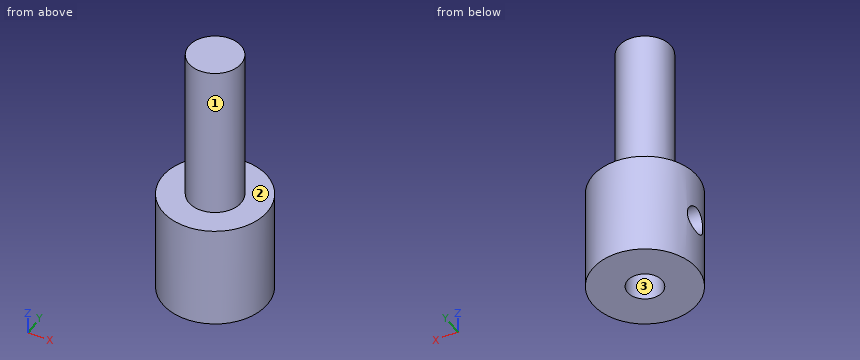
Autodesk Inventor part; units mm, degrees
ref_plane "YZ Plane" through (0, 0, 0) normal (1, 0, 0) x (0, 1, 0)
ref_plane "XZ Plane" through (0, 0, 0) normal (0, 1, 0) x (-1, 0, 0)
ref_plane "XY Plane" through (0, 0, 0) normal (0, 0, 1) x (1, 0, 0)
sketch "スケッチ1" plane through (0, 0, 0) normal (1, 0, 0) x (0, 1, 0)
  line L0 (0, 0) -> (1.5, 0)
  line L1 (1.5, 0) -> (1.5, -9)
  line L2 (1.5, -9) -> (3, -9)
  line L3 (3, -9) -> (3, -15)
  line L4 (3, -15) -> (1, -15)
  line L5 (0, 0) -> (0, -11)
  line L6 (0, -11) -> (1, -11)
  line L7 (1, -11) -> (1, -15)
  dimension "d0" = 1.5
  dimension "d1" = 1
  dimension "d2" = 9
  dimension "d3" = 4
  dimension "d4" = 2
  dimension "d5" = 2
revolve "回転1" add sketch "スケッチ1" angle 360 about axis through (0, 0, 0) along (0, 0, -1)
sketch "スケッチ2" plane through (0, 0, 0) normal (1, 0, 0) x (0, 1, 0)
  point P0 (0, 0)
  point P1 (0, -11.9211)
hole "穴1" at (0, 0, -11.9211) direction (-1, 0, 0) diameter 1.567 end through all
Design review of the part built by this model. Coordinates are the model's own, in mm. Face numbers are marked on the shaded views. Coordinates: 2 decimals unless noted, no trailing zeros. Order: outer loops, then holes, each group sorted by start corner. A loop starts at its lowest first (then second) coordinate and runs counter-clockwise, first axis right, second up.
Item 1: Take a section at C-C, the plane x = -1.25. Write out the cut boundary in (y, z), then the cut area to 3 significant figures.
Item 2: Take a section at B-B, the plane x = 0. Write out the cut boundary in (y, z), then the cut area to 3 significant figures.
Item 3: Take a section at A-A, the plane y = 0. Write out the cut boundary in (x, z), then the cut area to 3 significant figures.
Item 4: For line 1 (Z direction, x = -2.2, y = 0); line 2 (Z direction, x = -2, y = 1.25); line 3 (Z direction, x = -0.25, y = -0.25), list the stretches that pass through material, from the lowest coordinate up.
Item 5: Take a section at D-D, the plane z = -9.5. Write out the cut boundary in (x, y), then the cut area to 3 significant figures.
Item 6: For pin 1 Ø2 at (x, z) = (1, -5) entering from -Y; pin 2 Ø1 at (x, z) = (-0.5, -7) entering from +Y; pin 3 Ø1.5 at (y, z) = (-2, -2) entering from +X, all flat-tipped, find the tip position at first contact; note any pin that passes through.
Item 7: The part is to be moulded in two halves that separate along X. For the marked faces 1, 2 and 3, say which applies: pulls with the +X half, pulls with the -X half, needs draft (parallel to the pull), parting line crosses it, or undercut.
The answers:
1. outline: (-2.73, -15) - (2.73, -15) - (2.73, -9) - (0.83, -9) - (0.83, 0) - (-0.83, 0) - (-0.83, -9) - (-2.73, -9) - close; hole circle Ø1.57 at (0, -11.92)
1. area: 45.7 mm2
2. outline: (-3, -15) - (-1, -15) - (-1, -11) - (1, -11) - (1, -15) - (3, -15) - (3, -9) - (1.5, -9) - (1.5, 0) - (-1.5, 0) - (-1.5, -9) - (-3, -9) - close
2. area: 55.0 mm2
3. outline: (-3, -15) - (-1, -15) - (-1, -12.7) - (-3, -12.7) - close; (-3, -11.14) - (-1, -11.14) - (-1, -11) - (1, -11) - (1, -15) - (3, -15) - (3, -9) - (1.5, -9) - (1.5, 0) - (-1.5, 0) - (-1.5, -9) - (-3, -9) - close
3. area: 51.9 mm2
4. line 1: z = -15 to -12.7, -11.14 to -9
4. line 2: z = -15 to -9
4. line 3: z = -11 to 0
5. outline: circle Ø6 at (0, 0)
5. area: 28.3 mm2
6. pin 1: stops at y = -1.5
6. pin 2: stops at y = 1.5
6. pin 3: stops at x = 0.83
7. face 1: parting line crosses it
7. face 2: needs draft
7. face 3: undercut
